Geometry check sheet. Reference: the model listing, model coordinates, mm. A direction names the side the tool comes from. Round coordinates to 2 decimals unless told otherwise and drop trailing zeros. Order: outer loops, then holes, each group sorted by start corner. A loop starts at its lowest first (then second) coordinate and runs counter-clockwise, first axis right, second up.
```python
from build123d import *

# Parameters (mm, degrees)
F2_W     = 0.41187
F2_H     = 2.318905
F3_DEPTH = 12.5


with BuildPart() as f1:
    # F0 (on Front) → F1 (revolve)
    with BuildSketch(Plane.XZ):
        with BuildLine():
            Line((-2.5, -1), (-1.5, -1))
            Line((-1.5, -1), (-1.5, -6.928856))
            Line((-1.5, -6.928856), (-2.5, -6.928856))
            Line((-2.5, -6.928856), (-2.5, -39.004903))
            Line((-2.5, -39.004903), (0, -39.004903))
            Line((0, -39.004903), (0, 2.5))
            ThreePointArc((0, 2.5), (-1.767767, 1.767767), (-2.5, 0))
            Line((-2.5, 0), (-2.5, -1))
        make_face()
    revolve(axis=Axis((0, 0, -18.252452), (0, 0, -1)))

    # F2 (on Front) → F3 (cut, symmetric)
    with BuildSketch(Plane.XZ):
        with Locations((-0.205935, 2.348353)):
            Rectangle(F2_W, F2_H)
        with Locations((0.205935, 2.348353)):
            Rectangle(F2_W, F2_H)
    extrude(amount=F3_DEPTH, both=True, mode=Mode.SUBTRACT)


solid = f1.part
```
(1) Draft check along Z on faces 1 (the flat face through (0, 0, -39.005)), 2 (the flat face through (2, 0, -6.929)), 3 (the cylindrical face through (0.54, -2.44, -23.19)). Enter one of: released by +Z, released by -Z, zero draft, split by the parting line, or undercut.
Returned:
face 1: released by -Z
face 2: undercut
face 3: zero draft
(2) Depth check by flat-ended pin: P1, Ø1.4, axis at y = -1, z = 2, coming from the -X side; P2, Ø1.5, axis at x = 0.5, y = -1, coming from the +Z side; P3, Ø1.4, axis at y = 0.5, z = 1.5, coming from the +X side. Enter the tip coordinate at first touch or a pass-through.
Returned:
P1: stops at x = -1.97
P2: stops at z = 2.45
P3: stops at x = 2.34
(3) Sectioned sample at B-B, the plane z = -31. Record the cut outline in (x, y).
Returned:
outline: circle Ø5 at (0, 0)
(4) Sectioned sample at A-A, the plane z = -1.5. Record the cut outline in (x, y).
Returned:
outline: circle Ø3 at (0, 0)
(5) Material ranges on line 1 (Z direction, x = 0.1, y = -1.7); line 2 (Z direction, x = 0.15, y = -0.4); line 3 (Z direction, x = 1.4, y = 1.3), recorded low to high.
Returned:
line 1: z = -39 to -6.93, -1 to 1.19
line 2: z = -39 to 1.19
line 3: z = -39 to -6.93, -1 to 1.61
(6) Set-up check for faces 4 (the cylindrical face through (0.54, -2.44, -0.51)), 5 (the flat face through (0.412, 0, 2)), 6 (the cylindrical face through (1.5, 0.07, -4.01)): record each of +Z, -Z, +X, -X, +Y, -Y from which the full face is reachable in a straight line by a thin tool's end or side.
Returned:
face 4: +Z, -Z
face 5: +Z, +Y, -Y
face 6: none
